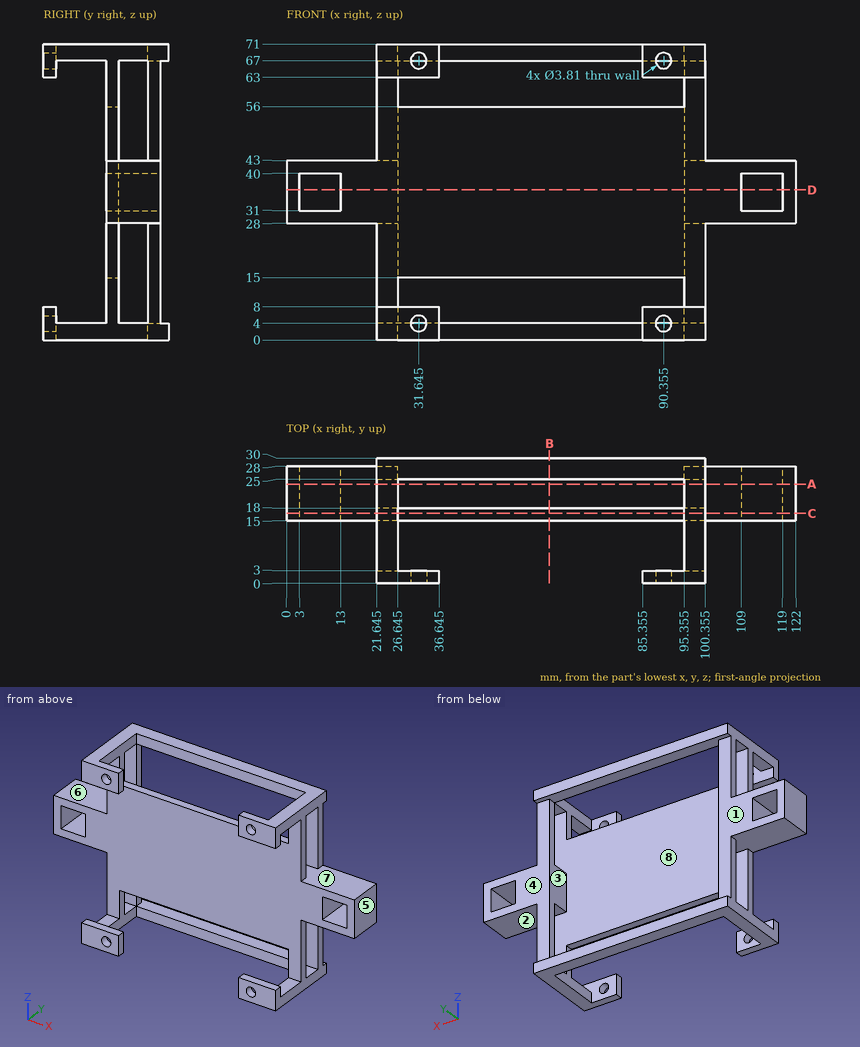
The figure shows three views and two pictorial views of one solid part (mm, origin at its lowest corner). Answer the questions. A direction names the side the tool comes from. Round coordinates to 2 decimals unless told otherwise and drop trailing zeros. Write each loop counter-clockwise with the first axis right and the second up, starting at its lowest first coordinate (ties: lowest second). Pieces come first, ordered by that corner, then holes. Notation, with made-up numbers: (-37.75, 47.5) -> (-21.75, 47.5) arc R12 ccw to (-21.75, 59.5) -> close; hole circle Ø10 at (63, 58). An arc over 180 degrees is marked (long way). Write each question's results on one line, items separated by ' | '.
Q1. Section C-C, the plane y = 16.75 is taken. Write down the section's boundary in (x, z) (3 decimals).
Data:
outline: (0, 28) -> (21.645, 28) -> (21.645, 0) -> (26.645, 0) -> (26.645, 15) -> (95.355, 15) -> (95.355, 0) -> (100.355, 0) -> (100.355, 28) -> (122, 28) -> (122, 43) -> (100.355, 43) -> (100.355, 71) -> (95.355, 71) -> (95.355, 56) -> (26.645, 56) -> (26.645, 71) -> (21.645, 71) -> (21.645, 43) -> (0, 43) -> close; hole (3, 31) -> (13, 31) -> (13, 40) -> (3, 40) -> close; hole (109, 31) -> (119, 31) -> (119, 40) -> (109, 40) -> close
Q2. Straight lines are drawn through the part: line 1 along X through (y, z) = (1.25, 67) (3 decimals); line 2 along X through (y, z) = (27.75, 39.5) (3 decimals); line 3 along Z through (x, y) = (6, 17.25). For each, find the intervals that lie inside material, in ascending order. Write a range as [from, to].
Data:
line 1: [21.645, 29.74], [33.55, 36.645], [85.355, 88.45], [92.26, 100.355] | line 2: [0, 3], [13, 26.645], [95.355, 109], [119, 122] | line 3: [28, 31], [40, 43]
Q3. Determine the mould class of the marked faces 1, 2 and 3 for opening direction Y: released by +Y, released by -Y, zero draft, split by the parting line, or undercut.
Data:
face 1: released by +Y | face 2: undercut | face 3: zero draft
Q4. Section A-A, the plane y = 23.75 is taken. Give the number of separate pieces and of enclosed holes in the cut face, then the cut area to 3 significant figures.
Data:
separate pieces: 6 | enclosed holes: 2 | area: 699 mm^2
Q5. Section D-D, the plane z = 36 is taken. Write down the section's boundary in (x, y) (3 decimals), then the cut area to 3 significant figures.
Data:
outline: (0, 15) -> (3, 15) -> (3, 28) -> (0, 28) -> close; (13, 15) -> (109, 15) -> (109, 28) -> (95.355, 28) -> (95.355, 18) -> (26.645, 18) -> (26.645, 28) -> (13, 28) -> close; (119, 15) -> (122, 15) -> (122, 28) -> (119, 28) -> close | area: 639 mm^2
Q6. Section B-B, the plane x = 63 is taken. Write down the section's boundary in (y, z), then the cut area to 3 significant figures.
Data:
outline: (15, 15) -> (18, 15) -> (18, 56) -> (15, 56) -> close; (25, 0) -> (30, 0) -> (30, 4) -> (25, 4) -> close; (25, 67) -> (30, 67) -> (30, 71) -> (25, 71) -> close | area: 163 mm^2
Q7. Flat-ended cylindrical pins translate along their axes: P1, Ø4, axis at y = 15.5, z = 43.5, coming from the -X side; P2, Ø6, axis at x = 85.5, y = 20, coming from the +Z side; P3, Ø2, axis at x = 87.5, y = 23, coming from the -Z side; P4, Ø2, axis at x = 16.5, y = 19.5, coming from the +Z side. Find the tip coordinate at first contact, or state that the pin passes through.
Data:
P1: x = 0 | P2: z = 56 | P3: through | P4: z = 43
Q8. Which of the six approach directions +Z, -Z, +X, -X, +Y, -Y give full straight-line access (tool end or side, diameter ignored) to the marked faces 4, 5, 6, 7 and 8?
Data:
face 4: +X, -X, +Y | face 5: +Z, -Z, +X, +Y, -Y | face 6: -X | face 7: +X | face 8: none
